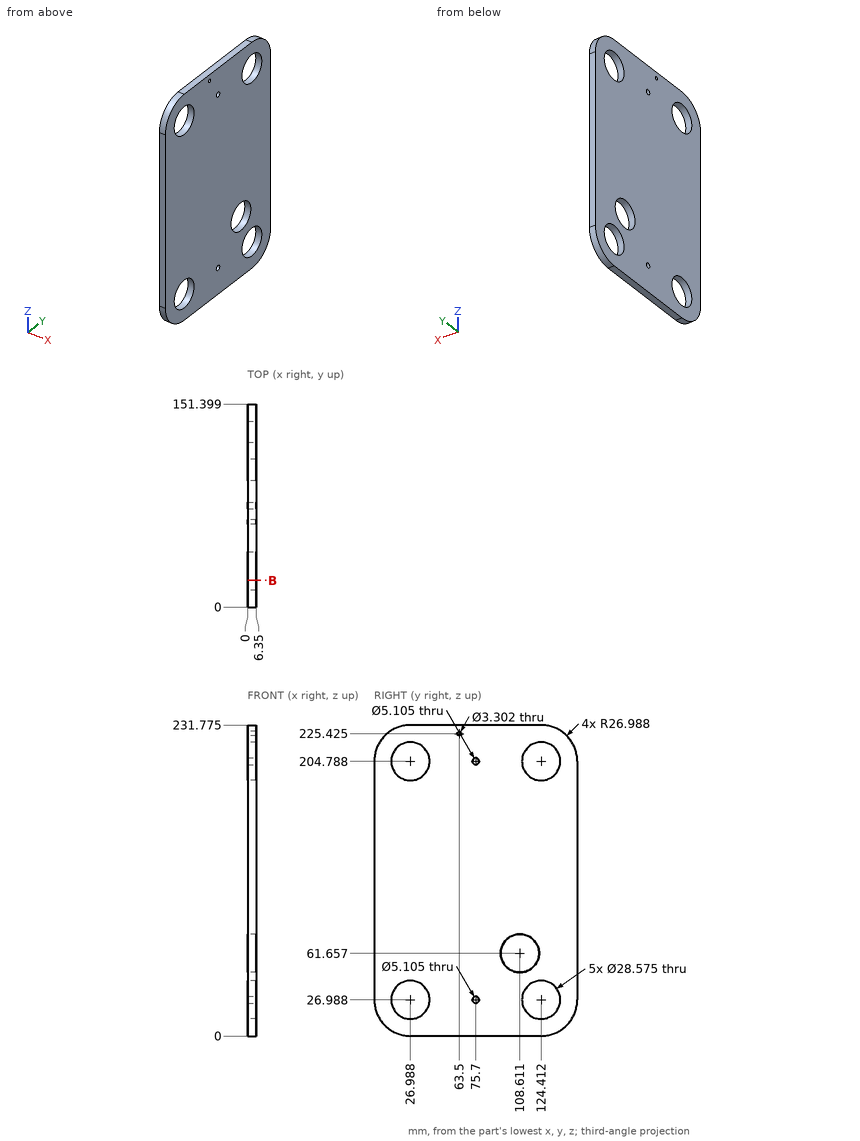
The figure shows three views and two pictorial views of one solid part (mm, origin at its lowest corner). Answer the questions. Give positions to 0.01 mm unless a question says otherwise; leave off trailing zeros. Answer in a Markdown table with one row per item.
(1) Consider L1, parallel to Z at x = 5.25, y = 76 (1 decimal); L2, parallel to Z at x = 0.5, y = 108.5 (1 decimal); L3, parallel to Z at x = 0.75, y = 30.5 (1 decimal). Determine where each line is inside the solid, lowest interval first. Write a range as [from, to].
Results list:
| item | result |
|---|---|
| L1 | z = [0, 24.5], [29.5, 202.3], [207.3, 231.8] |
| L2 | z = [0, 47.4], [75.9, 231.8] |
| L3 | z = [0, 13.1], [40.8, 190.9], [218.6, 231.8] |
(2) Section B-B (y = 20) is taken. State how many separate pieces and enclosed holes the cut face has, and give its area (3 significant figures).
Results list:
| item | result |
|---|---|
| separate pieces | 3 |
| enclosed holes | 0 |
| area | 1,140 mm² |
(3) A flat-ended cylindrical pin translates along its axis: pin 1 Ø3 at (y, z) = (75.7, 26.99) entering from -X. Find the tip coordinate at first contact, or state that the pin passes through.
Results list:
| item | result |
|---|---|
| pin 1 | passes through |
